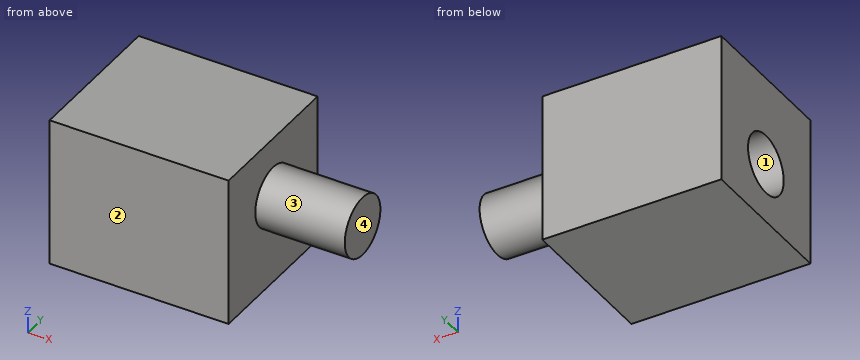
```python
from build123d import *

# Parameters (mm, degrees)
F0_W     = 60
F0_H     = 50
F1_DEPTH = 50
F2_R     = 10
F3_DEPTH = 30
F4_R     = 10
F5_DEPTH = 30


with BuildPart() as f1:
    # F0 (on Top) → F1 (new body)
    with BuildSketch(Plane.XY):
        Rectangle(F0_W, F0_H)
    extrude(amount=F1_DEPTH)

    # F2 (on face) → F3 (join)
    with BuildSketch(Plane.YZ.offset(30)):
        with Locations((0, 30)):
            Circle(F2_R)
    extrude(amount=F3_DEPTH)

    # F4 (on face) → F5 (cut)
    with BuildSketch(Plane(origin=(-30, 0, 0), x_dir=(0, -1, 0), z_dir=(-1, 0, 0))):
        with Locations((0, 20)):
            Circle(F4_R)
    extrude(amount=-F5_DEPTH, mode=Mode.SUBTRACT)


solid = f1.part
```
Geometry: final body of the model. Coordinates: model frame, mm. Face numbers are marked on the shaded views. Give positions to 0.01 mm unless a question says otherwise; leave off trailing zeros. Order: outer loops, then holes, each group sorted by start corner. A loop starts at its lowest first (then second) coordinate and runs counter-clockwise, first axis right, second up. Notation, with made-up numbers: (22, 30) -> (47, 30) arc R22 cw to (47, 56) -> close; hole circle Ø2 at (-25.5, -14.5). An arc over 180 degrees is marked (long way). Write each question's results on one line, items separated by ' | '. Start each with the question number.
1) Line query: line 1 (Z direction, x = -12, y = 0); line 2 (X direction, y = -6.5, z = 4); line 3 (Z direction, x = 52.5, y = 0). Output: solid intervals per line, ascending. Write a range as from..to.
2) Section D-D (x = 35.5). Return loops of the section in (y, z).
3) First-contact query: pin 1 (10 mm diameter, centred on y = 4.5, z = 21, fed in from -X); pin 2 (2 mm diameter, centred on x = 40.5, y = -12, fed in from +Z); pin 3 (1.5 mm diameter, centred on x = 34, y = 7.5, fed in from +Z). Flat tips, straight axial feed; report the tip coordinate or a pass-through.
4) Draft query along Y for the marked faces 1, 2, 3 and 4. Return one class per face: pulls with the +Y half, pulls with the -Y half, needs draft (parallel to the pull), parting line crosses it, or undercut.
5) Section B-B (z = 23.5). Return loops of the section in (x, y), then the cut area to 3 significant figures.
6) Section A-A (x = -19). Return loops of the section in (y, z), then the cut area to 3 significant figures.
7) Section C-C (y = 22.5). Return loops of the section in (x, z).
Calculated:
1) line 1: 0..10, 30..50 | line 2: -30..30 | line 3: 20..40
2) outline: circle Ø20 at (0, 30)
3) pin 1: x = 0 | pin 2: through | pin 3: z = 37.38
4) face 1: undercut | face 2: pulls with the -Y half | face 3: parting line crosses it | face 4: needs draft
5) outline: (-30, -25) -> (30, -25) -> (30, -7.6) -> (60, -7.6) -> (60, 7.6) -> (30, 7.6) -> (30, 25) -> (-30, 25) -> (-30, 9.37) -> (0, 9.37) -> (0, -9.37) -> (-30, -9.37) -> close | area: 2,890 mm2
6) outline: (-25, 0) -> (25, 0) -> (25, 50) -> (-25, 50) -> close; hole circle Ø20 at (0, 20) | area: 2,190 mm2
7) outline: (-30, 0) -> (30, 0) -> (30, 50) -> (-30, 50) -> close
